The model under review builds one solid part; all positions refer to its coordinate system, in mm. A direction names the side the tool comes from. Coordinates: 2 decimals unless noted, no trailing zeros. Loops run counter-clockwise (first coordinate to the right, second up) from the corner with the lowest first, then second, coordinate; pieces in that order, holes last. Notation, with made-up numbers: (-8, -2.75) - (3, -2.75) arc R30 ccw to (3, 35.25) - close; hole circle Ø8 at (48, -20). An arc over 180 degrees is marked (long way). Use a Markdown table: item, result. Add a question column.
1) To check wall thickness, follow L1, parallel to Z at x = 1.25, y = 11.5; L2, parallel to Z at x = -1.5, y = 72.5; L3, parallel to X at y = 60, z = -11. State the ranges of each line that lie inside material, in increasing order. Write a range as [from, to].
2) Add section C-C, the plane y = 64. Give the boundary of the cut face in (x, z), and give its area (3 significant figures).
3) Clearance check with flat-ended pins moving along their axes: pin 1 (10 mm diameter, centred on x = -28.5, z = -35, fed in from -Y); pin 2 (5.5 mm diameter, centred on x = -19.5, y = 10.5, fed in from +Z); pin 3 (4 mm diameter, centred on x = -2.5, z = -27, fed in from +Y); pin 4 (2 mm diameter, centred on y = 10, z = -17, fed in from -X). State where each tip first meets the part, or that it passes through.
4) Add section B-B, the plane x = -3. Give the boundary of the cut face in (y, z).
5) Add section D-D, the plane z = -21.5. Give the boundary of the cut face in (x, y), and give its area (3 significant figures).
6) For faces 1 (the flat face through (4.014, 12.894, -47.13)), 2 (the flat face through (-24, 10, -50)), 3 (the flat face through (-10, -4, -12.5)), 4 (the flat face through (-21, 10, -40)), list the 3-axis set-ups (+Z, -Z, +X, -X, +Y, -Y) from which the entire face can be reached by the end or side of a thin tool; tool diameter is ignored.
7) Add section A-A, the plane z = -27.5. Give the boundary of the cut face in (x, y).
8) The part is to be moulded in two halves that separate along X. For faces 5 (the cylindrical face through (-18.43, 11.06, -54.4)), 6 (the flat face through (0, 13, -30)), 7 (the flat face through (-24, 8, -8)), say which applies: pulls with the +X half, pulls with the -X half, needs draft (parallel to the pull), parting line crosses it, or undercut.
```python
from build123d import *

# Parameters (mm, degrees)
BOSS_EXTRUDE1_DEPTH     = 15
BOSS_EXTRUDE2_DEPTH     = 60
SKETCH3_W               = 24
SKETCH3_H               = 25
BOSS_EXTRUDE3_DEPTH     = 5
FILLET1_R               = 2
CUT_EXTRUDE1_DEPTH      = 109.374351209
CUT_EXTRUDE1_DEPTH_BACK = 9
SKETCH5_W               = 30
SKETCH5_H               = 12
CUT_EXTRUDE2_DEPTH      = 9
FILLET2_R               = 2
FILLET3_R               = 2
FILLET4_R               = 2
SKETCH6_W               = 15
SKETCH6_H               = 10
BOSS_EXTRUDE4_DEPTH     = 5
FILLET5_R               = 2
BOSS_EXTRUDE6_START     = 5
BOSS_EXTRUDE6_DEPTH     = 5
SKETCH11_R              = 1.75
CUT_EXTRUDE6_DEPTH      = 17
CUT_EXTRUDE7_DEPTH      = 2
SKETCH16_R              = 1.75
BOSS_EXTRUDE7_DEPTH     = 5
SKETCH17_W              = 5
SKETCH17_H              = 35
BOSS_EXTRUDE8_DEPTH     = 10
FILLET6_R               = 2


with BuildPart() as part:
    # Sketch1 → Boss-Extrude1 (new body)
    with BuildSketch(Plane.XY):
        with BuildLine():
            Line((0, 0), (0, 87))
            Line((0, 87), (-24, 87))
            Line((-24, 87), (-24, 67))
            Line((-24, 67), (-19, 67))
            Line((-19, 67), (-19, 80))
            ThreePointArc((-19, 80), (-18.414213562, 81.414213562), (-17, 82))
            Line((-17, 82), (-7, 82))
            ThreePointArc((-7, 82), (-5.585786438, 81.414213562), (-5, 80))
            Line((-5, 80), (-5, 75.913258959))
            Line((-5, 75.913258959), (-5, 0))
            Line((-5, 0), (0, 0))
        make_face()
    extrude(amount=-BOSS_EXTRUDE1_DEPTH)

    # Sketch2 → Boss-Extrude2 (add)
    with BuildSketch(Plane.XY):
        Polygon((-5, 0), (-24, 0), (-24, 0.85250732), (-24, 15), (-19, 15), (-19, 5), (-5, 5), (-5, 25), (0, 25), (0, 0), align=None)
    extrude(amount=-BOSS_EXTRUDE2_DEPTH)

    # Sketch3 → Boss-Extrude3 (add)
    with BuildSketch(Plane(origin=(0, 0, -60), x_dir=(-1, 0, 0), z_dir=(0, 0, -1))):
        with Locations((12, 12.5)):
            Rectangle(SKETCH3_W, SKETCH3_H)
    extrude(amount=-BOSS_EXTRUDE3_DEPTH)

    # Fillet1
    fillet1_edges = [part.edges().sort_by_distance(p)[0] for p in [
        (-5, 5, -27.5),
        (-19, 5, -27.5),
    ]]
    fillet(fillet1_edges, radius=FILLET1_R)

    # Sketch4 → Cut-Extrude1 (cut, two sides: drawn at the far end of the back side and taken through both)
    with BuildSketch(Plane.ZY.offset(24).offset(-CUT_EXTRUDE1_DEPTH_BACK)):
        Polygon((-55, 206.20706388), (-55, 15), (-55, 5), (-15, 5), (-15, 15), (-15, 206.20706388), (-15, 588.62119164), (-55, 588.62119164), align=None)
    extrude(amount=CUT_EXTRUDE1_DEPTH + CUT_EXTRUDE1_DEPTH_BACK, mode=Mode.SUBTRACT)

    # Sketch5 → Cut-Extrude2 (cut)
    with BuildSketch(Plane.ZY.offset(5)):
        with Locations((-30, 19)):
            Rectangle(SKETCH5_W, SKETCH5_H)
    extrude(amount=-CUT_EXTRUDE2_DEPTH, mode=Mode.SUBTRACT)

    # Fillet2
    fillet2_edges = [part.edges().sort_by_distance(p)[0] for p in [
        (-5, 16, -55),
        (-15.5, 5, -55),
        (-5.585786438, 5.585786438, -55),
    ]]
    fillet(fillet2_edges, radius=FILLET2_R)

    # Fillet3
    fillet3_edges = [part.edges().sort_by_distance(p)[0] for p in [
        (-2.5, 13, -45),
    ]]
    fillet(fillet3_edges, radius=FILLET3_R)

    # Fillet4
    fillet4_edges = [part.edges().sort_by_distance(p)[0] for p in [
        (-2.5, 13, -15),
    ]]
    fillet(fillet4_edges, radius=FILLET4_R)

    # Sketch6 → Boss-Extrude4 (add)
    with BuildSketch(Plane.ZY.offset(24)):
        with Locations((-47.5, 10)):
            Rectangle(SKETCH6_W, SKETCH6_H)
    extrude(amount=-BOSS_EXTRUDE4_DEPTH)

    # Fillet5
    fillet5_edges = [part.edges().sort_by_distance(p)[0] for p in [
        (-19, 5.585786438, -54.414213562),
        (-19, 11, -55),
        (-19, 5, -46.5),
    ]]
    fillet(fillet5_edges, radius=FILLET5_R)

    # Sketch10 → Boss-Extrude6 (add)
    with BuildSketch(Plane(origin=(0, 0, 0), x_dir=(0, 0, -1), z_dir=(1, 0, 0)).offset(BOSS_EXTRUDE6_START)):
        with BuildLine():
            Line((43, 13), (17, 13))
            ThreePointArc((17, 13), (15.585786438, 13.585786438), (15, 15))
            Line((15, 15), (15, 87))
            Line((15, 87), (0, 87))
            Line((0, 87), (0, 0))
            Line((0, 0), (60, 0))
            Line((60, 0), (60, 25))
            Line((60, 25), (45, 25))
            Line((45, 25), (45, 15))
            ThreePointArc((45, 15), (44.414213562, 13.585786438), (43, 13))
        make_face()
    extrude(amount=-BOSS_EXTRUDE6_DEPTH)

    # Sketch11 → Cut-Extrude6 (cut)
    with BuildSketch(Plane(origin=(5, 0, 0), x_dir=(0, 0, -1), z_dir=(1, 0, 0))):
        with Locations(Location((49.5, 11.5, 0), (0, 0, 90))):
            Circle(SKETCH11_R)
        with Locations(Location((7.248390946, 72.5, 0), (0, 0, 90))):
            Circle(SKETCH11_R)
    extrude(amount=-CUT_EXTRUDE6_DEPTH, mode=Mode.SUBTRACT)

    # Sketch14 → Cut-Extrude7 (cut)
    with BuildSketch(Plane(origin=(5, 0, 0), x_dir=(0, 0, -1), z_dir=(1, 0, 0))):
        Polygon((10.423817427, 72.5), (8.836104186, 75.25), (5.660677706, 75.25), (4.072964465, 72.5), (5.660677706, 69.75), (8.836104186, 69.75), align=None)
        Polygon((52.675426481, 11.5), (51.08771324, 14.25), (47.91228676, 14.25), (46.324573519, 11.5), (47.91228676, 8.75), (51.08771324, 8.75), align=None)
    extrude(amount=-CUT_EXTRUDE7_DEPTH, mode=Mode.SUBTRACT)

    # Sketch16 → Boss-Extrude7 (add)
    with BuildSketch(Plane(origin=(0, 0, 0), x_dir=(1, 0, 0), z_dir=(0, 1, 0))):
        with BuildLine():
            Line((-24, 35), (-41.5, 35))
            ThreePointArc((-41.5, 35), (-45.035533906, 33.535533906), (-46.5, 30))
            Line((-46.5, 30), (-46.5, 25))
            ThreePointArc((-46.5, 25), (-45.035533906, 21.464466094), (-41.5, 20))
            Line((-41.5, 20), (-24, 20))
            Line((-24, 20), (-24, 35))
        make_face()
        with Locations(Location((-42, 27.5, 0), (0, 0, 180))):
            Circle(SKETCH16_R, mode=Mode.SUBTRACT)
    extrude(amount=BOSS_EXTRUDE7_DEPTH)

    # Sketch17 → Boss-Extrude8 (add)
    with BuildSketch(Plane.XZ):
        with Locations((-9.5, -30)):
            Rectangle(SKETCH17_W, SKETCH17_H)
    extrude(amount=BOSS_EXTRUDE8_DEPTH)

    # Fillet6
    fillet6_edges = [part.edges().sort_by_distance(p)[0] for p in [
        (-9.5, -10, -12.5),
        (-9.5, -10, -47.5),
    ]]
    fillet(fillet6_edges, radius=FILLET6_R)


solid = part.part
```
From the geometry:
| question | item | result |
|---|---|---|
| 1 | L1 | z = [-60, -51.25], [-47.75, 0] |
| 1 | L2 | z = [-15, -9], [-5.5, 0] |
| 1 | L3 | x = [-5, 5] |
| 2 | outline | (-5, -15) - (5, -15) - (5, 0) - (-5, 0) - close |
| 2 | area | 150 mm^2 |
| 3 | pin 1 | stops at y = 0 |
| 3 | pin 2 | stops at z = 0 |
| 3 | pin 3 | stops at y = 13 |
| 3 | pin 4 | stops at x = -5 |
| 4 | outline | (0, -60) - (25, -60) - (25, -45) - (15, -45) arc R2 cw to (13, -43) - (13, -17) arc R2 cw to (15, -15) - (87, -15) - (87, 0) - (0, 0) - close; hole circle Ø3.5 at (11.5, -49.5); hole circle Ø3.5 at (72.5, -7.25) |
| 5 | outline | (-45.07, 0) - (-12, 0) - (-12, -10) - (-7, -10) - (-7, 0) - (5, 0) - (5, 13) - (-5, 13) - (-5, 7) arc R2 cw to (-7, 5) - (-45.07, 5) - close |
| 5 | area | 381 mm^2 |
| 6 | face 1 | +X |
| 6 | face 2 | -Z, -X, +Y, -Y |
| 6 | face 3 | +Z, +X, -X, -Y |
| 6 | face 4 | -X, +Y |
| 7 | outline | (-46.5, 0) - (-43.75, 0) - (-43.75, 5) - (-46.5, 5) - close; (-40.25, 0) - (-12, 0) - (-12, -10) - (-7, -10) - (-7, 0) - (5, 0) - (5, 13) - (-5, 13) - (-5, 7) arc R2 cw to (-7, 5) - (-40.25, 5) - close |
| 8 | face 5 | undercut |
| 8 | face 6 | needs draft |
| 8 | face 7 | pulls with the -X half |
